Here's how the part is built. I have some questions about the finished solid (model axes, mm). Face numbers are marked on the shaded views. Round coordinates to 2 decimals unless told otherwise and drop trailing zeros. Use a Markdown table: item, result.
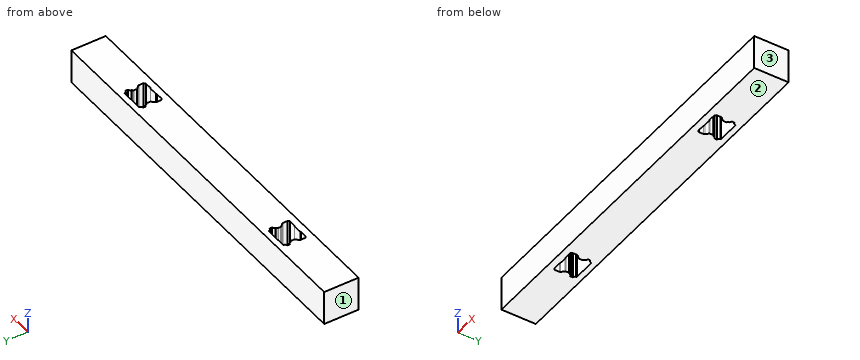
```python
from build123d import *

# Parameters (mm, degrees)
SKETCH_1_W      = 400
SKETCH_1_H      = 36
EXTRUDE_1_DEPTH = 36


with BuildPart() as part:
    # 草图1 → 凸台-拉伸1 (new body)
    with BuildSketch(Plane.XY):
        with Locations((146.804691074, 11.624598534)):
            Rectangle(SKETCH_1_W, SKETCH_1_H)
        with BuildLine():
            Line((18.304691074, 20.776588155), (18.304691074, 18.472608914))
            ThreePointArc((18.304691074, 18.472608914), (18.332858946, 18.345694397), (18.412073037, 18.242612627))
            ThreePointArc((18.412073037, 18.242612627), (19.826614478, 17.527140145), (20.52653516, 16.104839403))
            ThreePointArc((20.52653516, 16.104839403), (20.536242904, 16.093568263), (20.546497421, 16.082792187))
            Line((20.546497421, 16.082792187), (21.365351246, 15.263938362))
            ThreePointArc((21.365351246, 15.263938362), (21.690510372, 14.777303339), (21.804691074, 14.203278191))
            Line((21.804691074, 14.203278191), (21.804691074, 11.745724673))
            ThreePointArc((21.804691074, 11.745724673), (21.690473216, 11.171804017), (21.36535125, 10.685258701))
            Line((21.36535125, 10.685258701), (18.744030902, 8.063938362))
            ThreePointArc((18.744030902, 8.063938362), (18.418871775, 7.577303339), (18.304691074, 7.003278191))
            Line((18.304691074, 7.003278191), (18.304691074, 2.124598534))
            Line((18.304691074, 2.124598534), (19.804691074, 0.624598534))
            Line((19.804691074, 0.624598534), (27.304691074, 0.624598534))
            Line((27.304691074, 0.624598534), (27.804691074, 1.124598534))
            Line((27.804691074, 1.124598534), (36.804691074, 1.124598534))
            Line((36.804691074, 1.124598534), (37.304691074, 0.624598534))
            Line((37.304691074, 0.624598534), (44.804691074, 0.624598534))
            Line((44.804691074, 0.624598534), (46.304691074, 2.124598534))
            Line((46.304691074, 2.124598534), (46.304691074, 7.003472395))
            ThreePointArc((46.304691074, 7.003472395), (46.190473222, 7.577393054), (45.86535125, 8.063938367))
            Line((45.86535125, 8.063938367), (43.244030902, 10.685258706))
            ThreePointArc((43.244030902, 10.685258706), (42.918871775, 11.171893729), (42.804691074, 11.745918878))
            Line((42.804691074, 11.745918878), (42.804691075, 14.203500139))
            ThreePointArc((42.804691075, 14.203500139), (42.91891424, 14.777405867), (43.244030896, 15.263938368))
            Line((43.244030896, 15.263938368), (44.062884727, 16.082792187))
            ThreePointArc((44.062884727, 16.082792187), (44.073139243, 16.093568263), (44.082846988, 16.104839403))
            ThreePointArc((44.082846988, 16.104839403), (44.782767669, 17.527140145), (46.19730911, 18.242612627))
            ThreePointArc((46.19730911, 18.242612627), (46.276523201, 18.345694397), (46.304691074, 18.472608914))
            Line((46.304691074, 18.472608914), (46.304691074, 20.776588155))
            ThreePointArc((46.304691074, 20.776588155), (46.276523201, 20.903502671), (46.19730911, 21.006584442))
            ThreePointArc((46.19730911, 21.006584442), (44.782767669, 21.722056923), (44.082846988, 23.144357665))
            ThreePointArc((44.082846988, 23.144357665), (44.073139243, 23.155628805), (44.062884727, 23.166404881))
            Line((44.062884727, 23.166404881), (43.604691074, 23.624598534))
            Line((43.604691074, 23.624598534), (21.004691074, 23.624598534))
            Line((21.004691074, 23.624598534), (20.546497421, 23.166404881))
            ThreePointArc((20.546497421, 23.166404881), (20.536242905, 23.155628805), (20.52653516, 23.144357665))
            ThreePointArc((20.52653516, 23.144357665), (19.826614478, 21.722056923), (18.412073037, 21.006584442))
            ThreePointArc((18.412073037, 21.006584442), (18.332858946, 20.903502671), (18.304691074, 20.776588155))
        make_face(mode=Mode.SUBTRACT)
        with BuildLine():
            Line((246.304691074, 20.776588155), (246.304691074, 18.472608914))
            ThreePointArc((246.304691074, 18.472608914), (246.332858946, 18.345694397), (246.412073037, 18.242612627))
            ThreePointArc((246.412073037, 18.242612627), (247.826614478, 17.527140145), (248.52653516, 16.104839403))
            ThreePointArc((248.52653516, 16.104839403), (248.536242904, 16.093568263), (248.546497421, 16.082792187))
            Line((248.546497421, 16.082792187), (249.365351245, 15.263938362))
            ThreePointArc((249.365351245, 15.263938362), (249.690510372, 14.777303339), (249.804691074, 14.203278191))
            Line((249.804691074, 14.203278191), (249.804691074, 11.745724673))
            ThreePointArc((249.804691074, 11.745724673), (249.690473216, 11.171804017), (249.36535125, 10.685258701))
            Line((249.36535125, 10.685258701), (246.744030902, 8.063938362))
            ThreePointArc((246.744030902, 8.063938362), (246.418871775, 7.577303339), (246.304691074, 7.003278191))
            Line((246.304691074, 7.003278191), (246.304691074, 2.124598534))
            Line((246.304691074, 2.124598534), (247.804691074, 0.624598534))
            Line((247.804691074, 0.624598534), (255.304691074, 0.624598534))
            Line((255.304691074, 0.624598534), (255.804691074, 1.124598534))
            Line((255.804691074, 1.124598534), (264.804691074, 1.124598534))
            Line((264.804691074, 1.124598534), (265.304691074, 0.624598534))
            Line((265.304691074, 0.624598534), (272.804691074, 0.624598534))
            Line((272.804691074, 0.624598534), (274.304691074, 2.124598534))
            Line((274.304691074, 2.124598534), (274.304691074, 7.003472395))
            ThreePointArc((274.304691074, 7.003472395), (274.190473222, 7.577393054), (273.86535125, 8.063938367))
            Line((273.86535125, 8.063938367), (271.244030902, 10.685258706))
            ThreePointArc((271.244030902, 10.685258706), (270.918871775, 11.171893729), (270.804691074, 11.745918878))
            Line((270.804691074, 11.745918878), (270.804691074, 14.203500139))
            ThreePointArc((270.804691074, 14.203500139), (270.918914239, 14.777405867), (271.244030896, 15.263938368))
            Line((271.244030896, 15.263938368), (272.062884727, 16.082792187))
            ThreePointArc((272.062884727, 16.082792187), (272.073139243, 16.093568263), (272.082846987, 16.104839403))
            ThreePointArc((272.082846987, 16.104839403), (272.782767669, 17.527140145), (274.19730911, 18.242612627))
            ThreePointArc((274.19730911, 18.242612627), (274.276523201, 18.345694397), (274.304691074, 18.472608914))
            Line((274.304691074, 18.472608914), (274.304691074, 20.776588155))
            ThreePointArc((274.304691074, 20.776588155), (274.276523201, 20.903502671), (274.19730911, 21.006584442))
            ThreePointArc((274.19730911, 21.006584442), (272.782767669, 21.722056923), (272.082846987, 23.144357665))
            ThreePointArc((272.082846987, 23.144357665), (272.073139243, 23.155628805), (272.062884727, 23.166404881))
            Line((272.062884727, 23.166404881), (271.604691074, 23.624598534))
            Line((271.604691074, 23.624598534), (249.004691074, 23.624598534))
            Line((249.004691074, 23.624598534), (248.546497421, 23.166404881))
            ThreePointArc((248.546497421, 23.166404881), (248.536242905, 23.155628805), (248.52653516, 23.144357665))
            ThreePointArc((248.52653516, 23.144357665), (247.826614478, 21.722056923), (246.412073037, 21.006584442))
            ThreePointArc((246.412073037, 21.006584442), (246.332858946, 20.903502671), (246.304691074, 20.776588155))
        make_face(mode=Mode.SUBTRACT)
    extrude(amount=EXTRUDE_1_DEPTH)


solid = part.part
```
Q1. Imagine slicing it at A-A, the plane z = 28.5. Give the number of separate pieces and of enclosed holes in the cut face, then the cut area to 3 significant figures.
Return value:
| item | result |
|---|---|
| separate pieces | 1 |
| enclosed holes | 2 |
| area | 13,200 mm^2 |
Q2. We'd pull the mould along X, two halves only. Please class the marked faces 1, 2 and 3: pulls with the +X half, pulls with the -X half, needs draft (parallel to the pull), parting line crosses it, or undercut.
Return value:
| item | result |
|---|---|
| face 1 | pulls with the -X half |
| face 2 | needs draft |
| face 3 | pulls with the +X half |
Q3. I need wall thicknesses on line 1 (X direction, y = 13, z = 5); line 2 (X direction, y = 4, z = 11); line 3 (Y direction, x = 251.5, z = 6). Which ranges of each line are inside material? Lowest first, please. Write a range as from..to.
Return value:
| item | result |
|---|---|
| line 1 | x = -53.2..21.8, 42.8..249.8, 270.8..346.8 |
| line 2 | x = -53.2..18.3, 46.3..246.3, 274.3..346.8 |
| line 3 | y = -6.38..0.62, 23.62..29.62 |
